Here's how the part is built. I have some questions about the finished solid (model axes, mm). Round coordinates to 2 decimals unless told otherwise and drop trailing zeros. Loops run counter-clockwise (first coordinate to the right, second up) from the corner with the lowest first, then second, coordinate; pieces in that order, holes last. Notation, with made-up numbers: (9.25, 58) - (67.25, 58) arc R19 ccw to (67.25, 90) - close; hole circle Ø8 at (-21, 40). An arc over 180 degrees is marked (long way). Return JSON: item names as keys, results as strings. Group by question number.
```python
from build123d import *

# Parameters (mm, degrees)
SKETCH_1_W          = 103
SKETCH_1_H          = 67
EXTRUDE_1_DEPTH     = 3
SKETCH_2_R          = 1.55
SKETCH_2_R_2        = 1.5
CUT_EXTRUDE_1_DEPTH = 10
CUT_EXTRUDE_2_DEPTH = 10
FILLET_1_R          = 3
SKETCH_5_W          = 25.271228892
SKETCH_5_H          = 3
EXTRUDE_2_DEPTH     = 3
FILLET_2_R          = 3
CUT_EXTRUDE_3_DEPTH = 10
SKETCH_7_W          = 3
SKETCH_7_H          = 15
SKETCH_7_W_2        = 15
SKETCH_7_H_2        = 3
EXTRUDE_3_DEPTH     = 3
FILLET_3_R          = 2


with BuildPart() as part:
    # 草图1 → 凸台-拉伸1 (new body)
    with BuildSketch(Plane.XY):
        Rectangle(SKETCH_1_W, SKETCH_1_H)
    extrude(amount=EXTRUDE_1_DEPTH)

    # 草图2 → 切除-拉伸1 (cut)
    with BuildSketch(Plane.XY.offset(3)):
        with Locations((-18, 18)):
            Circle(SKETCH_2_R)
        with Locations((18, 18)):
            Circle(SKETCH_2_R)
        with Locations((18, -18)):
            Circle(SKETCH_2_R)
        with Locations((-18, -18)):
            Circle(SKETCH_2_R)
        with Locations((42.5, 29.7)):
            Circle(SKETCH_2_R_2)
        with Locations((42.5, -30.5)):
            Circle(SKETCH_2_R_2)
        with Locations((-42.499997562, -30.5)):
            Circle(SKETCH_2_R_2)
        with Locations((-42.499997562, 29.7)):
            Circle(SKETCH_2_R_2)
    extrude(amount=-CUT_EXTRUDE_1_DEPTH, mode=Mode.SUBTRACT)

    # 草图4 → 切除-拉伸2 (cut)
    with BuildSketch(Plane.XY.offset(3)):
        with BuildLine():
            Line((20.699726018, 20.951521544), (35.87816381, 28.2))
            Line((35.87816381, 28.2), (-35.878161967, 28.2))
            Line((-35.878161967, 28.2), (-20.699725904, 20.951521649))
            ThreePointArc((-20.699725904, 20.951521649), (-17.11629588, 21.901162266), (-14.291900756, 19.5))
            Line((-14.291900756, 19.5), (14.291900756, 19.5))
            ThreePointArc((14.291900756, 19.5), (17.116295955, 21.901162283), (20.699726018, 20.951521544))
        make_face()
        with BuildLine():
            Line((40.999997562, 27.321408738), (21.992528342, 18.244371513))
            ThreePointArc((21.992528342, 18.244371513), (21.383411469, 15.866334883), (19.5, 14.291900756))
            Line((19.5, 14.291900756), (19.5, -14.291900756))
            ThreePointArc((19.5, -14.291900756), (21.411123425, -15.910924372), (21.984738914, -18.349078486))
            Line((21.984738914, -18.349078486), (40.999997562, -28.050742027))
            Line((40.999997562, -28.050742027), (40.999997562, 27.321408738))
        make_face()
        with BuildLine():
            ThreePointArc((16.5, 14.291900756), (15.171572875, 15.171572875), (14.291900756, 16.5))
            Line((14.291900756, 16.5), (-14.291900756, 16.5))
            ThreePointArc((-14.291900756, 16.5), (-15.171572875, 15.171572875), (-16.5, 14.291900756))
            Line((-16.5, 14.291900756), (-16.5, -14.291900756))
            ThreePointArc((-16.5, -14.291900756), (-15.171572875, -15.171572875), (-14.291900756, -16.5))
            Line((-14.291900756, -16.5), (14.291900756, -16.5))
            ThreePointArc((14.291900756, -16.5), (15.171572875, -15.171572875), (16.5, -14.291900756))
            Line((16.5, -14.291900756), (16.5, 14.291900756))
        make_face()
        with BuildLine():
            ThreePointArc((-19.5, 14.291900756), (-21.383411469, 15.866334883), (-21.992528342, 18.244371513))
            Line((-21.992528342, 18.244371513), (-40.999997562, 27.321408738))
            Line((-40.999997562, 27.321408738), (-40.999997562, -28.050742027))
            Line((-40.999997562, -28.050742027), (-21.984738914, -18.349078486))
            ThreePointArc((-21.984738914, -18.349078486), (-21.411123425, -15.910924372), (-19.5, -14.291900756))
            Line((-19.5, -14.291900756), (-19.5, 14.291900756))
        make_face()
        with BuildLine():
            Line((35.87816381, -28.2), (20.699726018, -20.951521544))
            ThreePointArc((20.699726018, -20.951521544), (17.116295955, -21.901162283), (14.291900756, -19.5))
            Line((14.291900756, -19.5), (-14.291900756, -19.5))
            ThreePointArc((-14.291900756, -19.5), (-17.11629588, -21.901162266), (-20.699725904, -20.951521649))
            Line((-20.699725904, -20.951521649), (-35.878161967, -28.2))
            Line((-35.878161967, -28.2), (35.87816381, -28.2))
        make_face()
    extrude(amount=-CUT_EXTRUDE_2_DEPTH, mode=Mode.SUBTRACT)

    # 圆角1
    fillet_1_edges = [part.edges().sort_by_distance(p)[0] for p in [
        (16.5, -14.291900756, 1.5),
        (14.291900756, -16.5, 1.5),
        (-14.291900756, -16.5, 1.5),
        (-16.5, -14.291900756, 1.5),
        (-16.5, 14.291900756, 1.5),
        (-14.291900756, 16.5, 1.5),
        (14.291900756, 16.5, 1.5),
        (16.5, 14.291900756, 1.5),
        (14.291900756, -19.5, 1.5),
        (20.699726018, -20.951521544, 1.5),
        (35.87816381, -28.2, 1.5),
        (-35.878161967, -28.2, 1.5),
        (-20.699725904, -20.951521649, 1.5),
        (-14.291900756, -19.5, 1.5),
        (21.984738914, -18.349078486, 1.5),
        (19.5, -14.291900756, 1.5),
        (19.5, 14.291900756, 1.5),
        (21.992528342, 18.244371513, 1.5),
        (40.999997562, 27.321408738, 1.5),
        (40.999997562, -28.050742027, 1.5),
        (-19.5, -14.291900756, 1.5),
        (-21.984738914, -18.349078486, 1.5),
        (-40.999997562, -28.050742027, 1.5),
        (-40.999997562, 27.321408738, 1.5),
        (-21.992528342, 18.244371513, 1.5),
        (-19.5, 14.291900756, 1.5),
        (20.699726018, 20.951521544, 1.5),
        (14.291900756, 19.5, 1.5),
        (-14.291900756, 19.5, 1.5),
        (-20.699725904, 20.951521649, 1.5),
        (-35.878161967, 28.2, 1.5),
        (35.87816381, 28.2, 1.5),
    ]]
    fillet(fillet_1_edges, radius=FILLET_1_R)

    # 草图5 → 凸台-拉伸2 (add)
    with BuildSketch(Plane.XY.offset(3)):
        with Locations((-30.476283089, 0)):
            Rectangle(SKETCH_5_W, SKETCH_5_H)
        with Locations((30.476283089, 0)):
            Rectangle(SKETCH_5_W, SKETCH_5_H)
    extrude(amount=-EXTRUDE_2_DEPTH)

    # 圆角2
    fillet_2_edges = [part.edges().sort_by_distance(p)[0] for p in [
        (-19.5, -1.5, 1.5),
        (-19.5, 1.5, 1.5),
        (-40.999997562, 1.5, 1.5),
        (-40.999997562, -1.5, 1.5),
        (40.999997562, -1.5, 1.5),
        (40.999997562, 1.5, 1.5),
        (19.5, 1.5, 1.5),
        (19.5, -1.5, 1.5),
        (-51.5, 33.5, 1.5),
        (51.5, 33.5, 1.5),
        (51.5, -33.5, 1.5),
        (-51.5, -33.5, 1.5),
    ]]
    fillet(fillet_2_edges, radius=FILLET_2_R)

    # 草图6 → 切除-拉伸3 (cut)
    with BuildSketch(Plane.XY.offset(3)):
        with BuildLine():
            Line((-42.999997562, 23.7), (-42.999997562, 6))
            ThreePointArc((-42.999997562, 6), (-46.249998781, 2.749998781), (-49.5, 6))
            Line((-49.5, 6), (-49.5, 23.7))
            ThreePointArc((-49.5, 23.7), (-46.249998781, 26.950001219), (-42.999997562, 23.7))
        make_face()
        with BuildLine():
            Line((42.999997562, 23.7), (42.999997562, 6))
            ThreePointArc((42.999997562, 6), (46.249998781, 2.749998781), (49.5, 6))
            Line((49.5, 6), (49.5, 23.7))
            ThreePointArc((49.5, 23.7), (46.249998781, 26.950001219), (42.999997562, 23.7))
        make_face()
        with BuildLine():
            Line((42.999997562, -23.7), (42.999997562, -6))
            ThreePointArc((42.999997562, -6), (46.249998781, -2.749998781), (49.5, -6))
            Line((49.5, -6), (49.5, -23.7))
            ThreePointArc((49.5, -23.7), (46.249998781, -26.950001219), (42.999997562, -23.7))
        make_face()
        with BuildLine():
            Line((-42.999997562, -23.7), (-42.999997562, -6))
            ThreePointArc((-42.999997562, -6), (-46.249998781, -2.749998781), (-49.5, -6))
            Line((-49.5, -6), (-49.5, -23.7))
            ThreePointArc((-49.5, -23.7), (-46.249998781, -26.950001219), (-42.999997562, -23.7))
        make_face()
    extrude(amount=-CUT_EXTRUDE_3_DEPTH, mode=Mode.SUBTRACT)

    # 草图7 → 凸台-拉伸3 (add)
    with BuildSketch(Plane.XY.offset(3)):
        with Locations((0, 9)):
            Rectangle(SKETCH_7_W, SKETCH_7_H)
        with Locations((-9, 0)):
            Rectangle(SKETCH_7_W_2, SKETCH_7_H_2)
        Rectangle(SKETCH_7_W, SKETCH_7_H_2)
        with Locations((9, 0)):
            Rectangle(SKETCH_7_W_2, SKETCH_7_H_2)
        with Locations((0, -9)):
            Rectangle(SKETCH_7_W, SKETCH_7_H)
    extrude(amount=-EXTRUDE_3_DEPTH)

    # 圆角3
    fillet_3_edges = [part.edges().sort_by_distance(p)[0] for p in [
        (1.5, 16.5, 1.5),
        (1.5, 1.5, 1.5),
        (16.5, 1.5, 1.5),
        (16.5, -1.5, 1.5),
        (1.5, -1.5, 1.5),
        (1.5, -16.5, 1.5),
        (-1.5, -16.5, 1.5),
        (-1.5, -1.5, 1.5),
        (-16.5, -1.5, 1.5),
        (-16.5, 1.5, 1.5),
        (-1.5, 1.5, 1.5),
        (-1.5, 16.5, 1.5),
    ]]
    fillet(fillet_3_edges, radius=FILLET_3_R)


solid = part.part
```
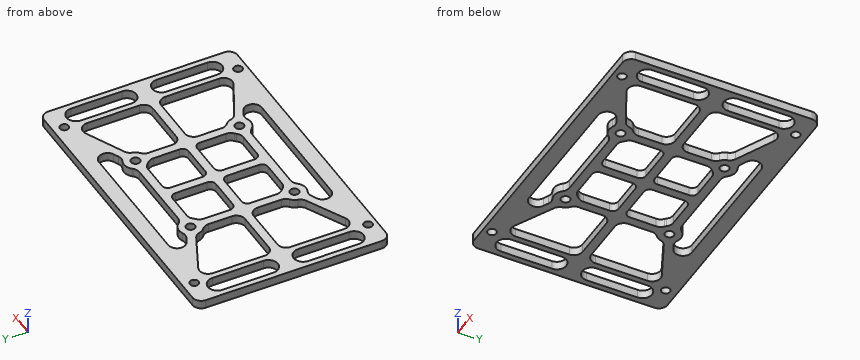
Q1. Imagine slicing it at D-D, the plane x = 17.5. List the corners of the cut face in (y, z) for me, and give its area (3 significant figures).
Q2. Imagine slicing it at B-B, the plane x = -11. List the corners of the cut face in (y, z) for me.
Q3. Imagine slicing it at C-C, the plane x = 33.5. List the corners of the cut face in (y, z) for me.
Q4. Imagine slicing it at A-A, the plane y = 11. List the corners of the cut face in (x, z) for me.
Q5. Please list where these lines run through material, in increasing order: line 1 (Y direction, x = -7, z = 0.3); line 2 (Y direction, x = -18, z = 0.85); line 3 (X direction, y = -23.5, z = 2.65).
Output values:
{
 "1": {"outline": "(-33.5, 0) - (-28.2, 0) - (-28.2, 3) - (-33.5, 3) - close; (-21.97, 0) - (-19.47, 0) - (-19.47, 3) - (-21.97, 3) - close; (-16.53, 0) - (16.53, 0) - (16.53, 3) - (-16.53, 3) - close; (19.47, 0) - (21.97, 0) - (21.97, 3) - (19.47, 3) - close; (28.2, 0) - (33.5, 0) - (33.5, 3) - (28.2, 3) - close", "area": "146 mm^2"},
 "2": {"outline": "(-33.5, 0) - (-28.2, 0) - (-28.2, 3) - (-33.5, 3) - close; (-19.5, 0) - (-16.5, 0) - (-16.5, 3) - (-19.5, 3) - close; (-1.5, 0) - (1.5, 0) - (1.5, 3) - (-1.5, 3) - close; (16.5, 0) - (19.5, 0) - (19.5, 3) - (16.5, 3) - close; (28.2, 0) - (33.5, 0) - (33.5, 3) - (28.2, 3) - close"},
 "3": {"outline": "(-33.5, 0) - (-24.22, 0) - (-24.22, 3) - (-33.5, 3) - close; (-1.5, 0) - (1.5, 0) - (1.5, 3) - (-1.5, 3) - close; (23.74, 0) - (33.5, 0) - (33.5, 3) - (23.74, 3) - close"},
 "4": {"outline": "(-51.5, 0) - (-49.5, 0) - (-49.5, 3) - (-51.5, 3) - close; (-43, 0) - (-41, 0) - (-41, 3) - (-43, 3) - close; (-19.5, 0) - (-16.5, 0) - (-16.5, 3) - (-19.5, 3) - close; (-1.5, 0) - (1.5, 0) - (1.5, 3) - (-1.5, 3) - close; (16.5, 0) - (19.5, 0) - (19.5, 3) - (16.5, 3) - close; (41, 0) - (43, 0) - (43, 3) - (41, 3) - close; (49.5, 0) - (51.5, 0) - (51.5, 3) - (49.5, 3) - close"},
 "5": {"line 1": "y = -33.5 to -28.2, -19.5 to -16.5, -1.5 to 1.5, 16.5 to 19.5, 28.2 to 33.5", "line 2": "y = -33.5 to -28.2, -22 to -19.55, -16.45 to 16.45, 19.55 to 22, 28.2 to 33.5", "line 3": "x = -51.5 to -49.5, -43 to -40.98, -32.08 to -25.11, 25.11 to 32.08, 40.98 to 43, 49.5 to 51.5"}
}
